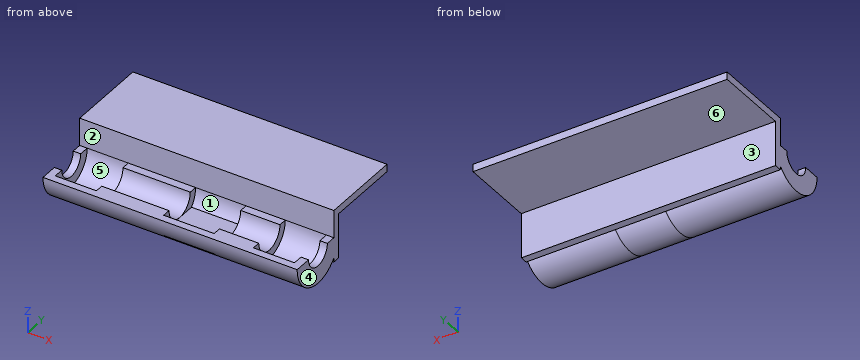
```python
from build123d import *

# Parameters (mm, degrees)
F0_W      = 340
F0_H      = 70
F1_DEPTH  = 10
F2_W      = 340
F2_H      = 100
F3_DEPTH  = 10
F7_ANGLE  = 180
F8_R      = 19.5
F9_DEPTH  = 170.001
F10_DEPTH = 170.001
F12_W     = 67.5
F12_H     = 66
F13_DEPTH = 25
F15_DEPTH = 222.501


with BuildPart() as f1:
    # F0 (on Front) → F1 (new body)
    with BuildSketch(Plane.XZ):
        with Locations((0, -25)):
            Rectangle(F0_W, F0_H)
    extrude(amount=F1_DEPTH)

    # F2 (on Top) → F3 (join)
    with BuildSketch(Plane.XY):
        with Locations((0, 50)):
            Rectangle(F2_W, F2_H)
    extrude(amount=F3_DEPTH)

    # F5 (on offset) → F7 (revolve)
    with BuildSketch(Plane.XY.offset(-27)):
        Polygon((170, 0), (-170, 0), (-170, -43), (-160, -43), (-160, -10), (-105, -10), (-105, -21), (-15, -21), (-15, -10), (52.5, -10), (52.5, -21), (105, -21), (105, -10), (160, -10), (160, -43), (170, -43), align=None)
    revolve(axis=Axis((0, -43, -27), (-1, 0, 0)), revolution_arc=F7_ANGLE)

    # F8 (on Right) → F9 (cut, through all)
    with BuildSketch(Plane.YZ):
        with Locations((-43, -27)):
            Circle(F8_R)
    extrude(amount=F9_DEPTH, mode=Mode.SUBTRACT)

    # F8 (on Right) → F10 (cut, through all)
    with BuildSketch(Plane.YZ):
        with Locations((-43, -27)):
            Circle(F8_R)
    extrude(amount=-F10_DEPTH, mode=Mode.SUBTRACT)

    # F12 (on offset) → F13 (join)
    with BuildSketch(Plane.XY.offset(-49)):
        with Locations((18.75, -43)):
            Rectangle(F12_W, F12_H)
    extrude(amount=-F13_DEPTH)

    # F14 (on face) → F15 (cut, through all)
    with BuildSketch(Plane.YZ.offset(52.5)):
        with BuildLine():
            ThreePointArc((-10, -54.568098), (-43, -70), (-76, -54.568098))
            Line((-76, -54.568098), (-76, -74))
            Line((-76, -74), (-10, -74))
            Line((-10, -74), (-10, -54.568098))
        make_face()
    extrude(amount=-F15_DEPTH, mode=Mode.SUBTRACT)


solid = f1.part
```
Verification items for the finished model (mm, model axes). Face numbers are marked on the shaded views. A direction names the side the tool comes from. Coordinates: 2 decimals unless noted, no trailing zeros. Loops run counter-clockwise (first coordinate to the right, second up) from the corner with the lowest first, then second, coordinate; pieces in that order, holes last. Notation, with made-up numbers: (71, 59.25) - (123, 59.25) arc R29 cw to (123, 90.25) - close; hole circle Ø8 at (31.25, 27.25). An arc over 180 degrees is marked (long way). Return JSON: item names as keys, results as strings.
1. Go/stop test with flat-tipped pins: pin 1 (5 mm diameter, centred on x = 6.5, y = -6, fed in from -Z); pin 2 (12 mm diameter, centred on x = -112, y = 53.5, fed in from -Z); pin 3 (1.6 mm diameter, centred on x = 76.5, z = -56, fed in from -Y); pin 4 (10 mm diameter, centred on y = -25.5, z = -21.5, fed in from +X). Record where each tip stops, or that it passes through.
Established:
{"pin 1": "stops at z = -60", "pin 2": "stops at z = 0", "pin 3": "stops at y = -75.46", "pin 4": "passes through"}
2. Thickness scan on L1, parallel to Y at x = 73, z = -28.5; L2, parallel to Y at x = 34.5, z = -27.5; L3, parallel to Y at x = 131, z = -3. Record the ranges inside material, lowest first.
Established:
{"L1": "y = -85.97 to -64.95, -21.05 to 0", "L2": "y = -86 to -76, -10 to 0", "L3": "y = -10 to 0"}
3. Tool access check on the marked faces 4, 5 and 6. Record the directions out of +Z, -Z, +X, -X, +Y, -Y that give a thin tool (end or side, any length) a straight path to the whole face; none if there is none.
Established:
{"face 4": "+Z, -Z, +X, +Y, -Y", "face 5": "+Z", "face 6": "-Z, +X, -X, +Y"}
4. Section check A-A, the plane x = -47.5. Record the boundary of the cut face in (y, z).
Established:
{"outline": "(-86, -27) arc R43 ccw to (-10, -54.57) - (-10, -60) - (0, -60) - (0, 0) - (100, 0) - (100, 10) - (-10, 10) - (-10, -27) - (-21, -27) arc R22 cw to (-65, -27) - close"}
5. Section check B-B, the plane y = -51.5. Record the boundary of the cut face in (x, z).
Established:
{"outline": "(-170, -69.15) - (170, -69.15) - (170, -44.55) - (160, -44.55) - (160, -58.89) - (105, -58.89) - (105, -47.29) - (52.5, -47.29) - (52.5, -49) - (-15, -49) - (-15, -47.29) - (-105, -47.29) - (-105, -58.89) - (-160, -58.89) - (-160, -44.55) - (-170, -44.55) - close"}
6. Section check D-D, the plane y = 21. Record the boundary of the cut face in (x, z), then the cut area to 3 significant figures.
Established:
{"outline": "(-170, 0) - (170, 0) - (170, 10) - (-170, 10) - close", "area": "3,400 mm2"}
7. Section check C-C, the plane x = 13. Record the boundary of the cut face in (y, z), then the cut area to 3 significant figures.
Established:
{"outline": "(-86, -27) arc R43 ccw to (-10, -54.57) - (-10, -60) - (0, -60) - (0, 0) - (100, 0) - (100, 10) - (-10, 10) - (-10, -27) arc R33 cw to (-18.4, -49) - (-67.6, -49) arc R33 cw to (-76, -27) - close", "area": "3,080 mm2"}
8. Mould release check, pull along Y, two halves, no side actions. Record for the marked faces 1, 2 and 3: +Y half, -Y half, draft (parallel to the pull), parting line (faces both ways), or undercut.
Established:
{"face 1": "undercut", "face 2": "-Y half", "face 3": "+Y half"}
